Build history of the part. All positions in model axes, mm. Give positions to 0.01 mm unless a question says otherwise; leave off trailing zeros. Write each loop counter-clockwise with the first axis right and the second up, starting at its lowest first coordinate (ties: lowest second). Pieces come first, ordered by that corner, then holes. Notation, with made-up numbers: (16, 64.5) -> (69, 64.5) arc R23 cw to (69, 88.5) -> close; hole circle Ø3 at (-35, 38). An arc over 180 degrees is marked (long way). One line per question, with ' | ' between items. Start each with the question number.
(1) Band-saw the part on A-A, the plane y = -23. Give the cut face in (x, z), and give its area (3 significant figures).
(2) Band-saw the part on B-B, the plane x = -35. Give the cut face in (y, z).
(3) Band-saw the part on D-D, the plane x = -2.5. Give the cut face in (y, z).
(4) Drill centre lines: probe 1 along X at (y, z) = (-30, 0.9); probe 2 along X at (y, z) = (-3, 3.25); probe 3 along Y at (x, z) = (42.5, 3.6). Where is each one in solid material? Low to high. Write a range as from..to.
(5) Band-saw the part on C-C, the plane z = 3. Count the separate pieces of the cut face and the enclosed holes in it, and give its area (3 significant figures).
from build123d import *

# Parameters (mm, degrees)
SKETCH1_R           = 2.1
BOSS_EXTRUDE1_DEPTH = 5
CUT_EXTRUDE1_DEPTH  = 5
SKETCH3_W           = 38.251438616
SKETCH3_H           = 32.766065525
CUT_EXTRUDE2_DEPTH  = 10
BOSS_EXTRUDE2_DEPTH = 5
SKETCH5_W           = 101.856885825
SKETCH5_H           = 15.226385752
CUT_EXTRUDE3_DEPTH  = 10
BOSS_EXTRUDE3_DEPTH = 5
CUT_EXTRUDE4_DEPTH  = 5
SKETCH8_R           = 2.5
SKETCH8_W           = 20
SKETCH8_H           = 40
CUT_EXTRUDE5_DEPTH  = 5
FILLET2_R           = 7


with BuildPart() as part:
    # Sketch1 → Boss-Extrude1 (new body)
    with BuildSketch(Plane.XY):
        Polygon((27.058043777, 13.348752177), (18.058043777, 13.348752177), (18.058043777, 18.348752177), (-18.941956223, 18.348752177), (-18.941956223, 13.348752177), (-27.941956223, 13.348752177), (-27.941956223, 1.348752177), (-27.941956223, -10.651247823), (-63.297295282, -46.006586882), (-51.297295282, -58.006586882), (50.413382836, -58.006586882), (62.413382836, -46.006586882), (27.058043777, -10.651247823), (27.058043777, 1.348752177), align=None)
        with Locations((9.558043777, -11.651247823)):
            Circle(SKETCH1_R, mode=Mode.SUBTRACT)
        with Locations((-10.441956223, -11.651247823)):
            Circle(SKETCH1_R, mode=Mode.SUBTRACT)
        with Locations((-10.441956223, 14.348752177)):
            Circle(SKETCH1_R, mode=Mode.SUBTRACT)
        with Locations((9.558043777, 14.348752177)):
            Circle(SKETCH1_R, mode=Mode.SUBTRACT)
        with BuildLine():
            ThreePointArc((-8.691956223, 1.348752177), (-12.941956223, 5.598752177), (-17.191956223, 1.348752177))
            ThreePointArc((-17.191956223, 1.348752177), (-12.941956223, -2.901247823), (-8.691956223, 1.348752177))
        make_face(mode=Mode.SUBTRACT)
        with BuildLine():
            ThreePointArc((16.308043777, 1.348752177), (12.058043777, 5.598752177), (7.808043777, 1.348752177))
            ThreePointArc((7.808043777, 1.348752177), (12.058043777, -2.901247823), (16.308043777, 1.348752177))
        make_face(mode=Mode.SUBTRACT)
    extrude(amount=BOSS_EXTRUDE1_DEPTH)

    # Sketch2 → Cut-Extrude1 (cut)
    with BuildSketch(Plane(origin=(0, 0, 0), x_dir=(-1, 0, 0), z_dir=(0, 0, -1))):
        with BuildLine():
            Line((-27.058043777, -22.48694002), (-27.058043777, -151.230871916))
            ThreePointArc((-27.058043777, -151.230871916), (0.441956223, -156.858905968), (27.941956223, -151.230871916))
            Line((27.941956223, -151.230871916), (27.941956223, -22.48694002))
            ThreePointArc((27.941956223, -22.48694002), (0.441956223, -16.858905968), (-27.058043777, -22.48694002))
        make_face()
    extrude(amount=-CUT_EXTRUDE1_DEPTH, mode=Mode.SUBTRACT)

    # Sketch3 → Cut-Extrude2 (cut)
    with BuildSketch(Plane(origin=(0, 0, 0), x_dir=(-1, 0, 0), z_dir=(0, 0, -1))):
        with Locations((-46.183763085, -43.921177391)):
            Rectangle(SKETCH3_W, SKETCH3_H)
        with Locations((47.067675531, -43.921177391)):
            Rectangle(SKETCH3_W, SKETCH3_H)
    extrude(amount=-CUT_EXTRUDE2_DEPTH, mode=Mode.SUBTRACT)

    # Sketch4 → Boss-Extrude2 (add)
    with BuildSketch(Plane(origin=(0, 0, 0), x_dir=(-1, 0, 0), z_dir=(0, 0, -1))):
        with BuildLine():
            Line((27.941956223, -10.651247823), (44.828853028, -27.538144628))
            Line((44.828853028, -27.538144628), (50.941956223, -27.538144628))
            Line((50.941956223, -27.538144628), (50.941956223, 27.461855372))
            ThreePointArc((50.941956223, 27.461855372), (49.477490129, 30.997389278), (45.941956223, 32.461855372))
            Line((45.941956223, 32.461855372), (-45.058043777, 32.461855372))
            ThreePointArc((-45.058043777, 32.461855372), (-48.593577683, 30.997389278), (-50.058043777, 27.461855372))
            Line((-50.058043777, 27.461855372), (-50.058043777, -27.538144628))
            Line((-50.058043777, -27.538144628), (-43.944940582, -27.538144628))
            Line((-43.944940582, -27.538144628), (-27.058043777, -10.651247823))
            Line((-27.058043777, -10.651247823), (-27.058043777, 13.348752177))
            Line((-27.058043777, 13.348752177), (-18.058043777, 13.348752177))
            Line((-18.058043777, 13.348752177), (-18.058043777, 18.348752177))
            Line((-18.058043777, 18.348752177), (18.941956223, 18.348752177))
            Line((18.941956223, 18.348752177), (18.941956223, 13.348752177))
            Line((18.941956223, 13.348752177), (27.941956223, 13.348752177))
            Line((27.941956223, 13.348752177), (27.941956223, -10.651247823))
        make_face()
    extrude(amount=-BOSS_EXTRUDE2_DEPTH)

    # Sketch5 → Cut-Extrude3 (cut)
    with BuildSketch(Plane.XY.offset(5)):
        with Locations((-0.013513311, 25.961945053)):
            Rectangle(SKETCH5_W, SKETCH5_H)
    extrude(amount=-CUT_EXTRUDE3_DEPTH, mode=Mode.SUBTRACT)

    # Sketch6 → Boss-Extrude3 (add)
    with BuildSketch(Plane.XY.offset(5)):
        with BuildLine():
            Line((50.058043777, -27.538144628), (27.058043777, -27.538144628))
            Line((27.058043777, -27.538144628), (27.058043777, -22.48694002))
            ThreePointArc((27.058043777, -22.48694002), (-0.441956223, -16.858905968), (-27.941956223, -22.48694002))
            Line((-27.941956223, -22.48694002), (-27.941956223, -27.538144628))
            Line((-27.941956223, -27.538144628), (-50.941956223, -27.538144628))
            Line((-50.941956223, -27.538144628), (-50.941956223, -42.538144628))
            Line((-50.941956223, -42.538144628), (-12.941956223, -42.538144628))
            Line((-12.941956223, -42.538144628), (12.058043777, -42.538144628))
            Line((12.058043777, -42.538144628), (50.058043777, -42.538144628))
            Line((50.058043777, -42.538144628), (50.058043777, -27.538144628))
        make_face()
    extrude(amount=-BOSS_EXTRUDE3_DEPTH)

    # Sketch7 → Cut-Extrude4 (cut)
    with BuildSketch(Plane.XY.offset(5)):
        with BuildLine():
            Line((-27.941956223, -27.962811021), (-27.941956223, -42.538144628))
            Line((-27.941956223, -42.538144628), (27.058043777, -42.538144628))
            Line((27.058043777, -42.538144628), (27.058043777, -27.962811021))
            ThreePointArc((27.058043777, -27.962811021), (-0.441956223, -21.858905968), (-27.941956223, -27.962811021))
        make_face()
    extrude(amount=-CUT_EXTRUDE4_DEPTH, mode=Mode.SUBTRACT)

    # Sketch8 → Cut-Extrude5 (cut)
    with BuildSketch(Plane(origin=(0, 0, 0), x_dir=(-1, 0, 0), z_dir=(0, 0, -1))):
        with Locations((44.521956223, 12.405303775)):
            Circle(SKETCH8_R)
        with Locations((34.361956223, 12.405303775)):
            Circle(SKETCH8_R)
        with Locations((34.361956223, -36.594696225)):
            Circle(SKETCH8_R)
        with Locations((44.521956223, -36.594696225)):
            Circle(SKETCH8_R)
        with Locations((-43.638043777, -36.594696225)):
            Circle(SKETCH8_R)
        with Locations((-33.478043777, -36.594696225)):
            Circle(SKETCH8_R)
        with Locations((-33.478043777, 12.405303775)):
            Circle(SKETCH8_R)
        with Locations((-43.638043777, 12.405303775)):
            Circle(SKETCH8_R)
        with Locations((39.441956223, -12.094696225)):
            Rectangle(SKETCH8_W, SKETCH8_H)
        with Locations((-38.558043777, -12.094696225)):
            Rectangle(SKETCH8_W, SKETCH8_H)
    extrude(amount=-CUT_EXTRUDE5_DEPTH, mode=Mode.SUBTRACT)

    # Fillet2
    fillet2_edges = [part.edges().sort_by_distance(p)[0] for p in [
        (50.058043777, 18.348752177, 2.5),
        (-50.941956223, 18.348752177, 2.5),
        (50.058043777, -42.538144628, 2.5),
        (-50.941956223, -42.538144628, 2.5),
    ]]
    fillet(fillet2_edges, radius=FILLET2_R)


solid = part.part
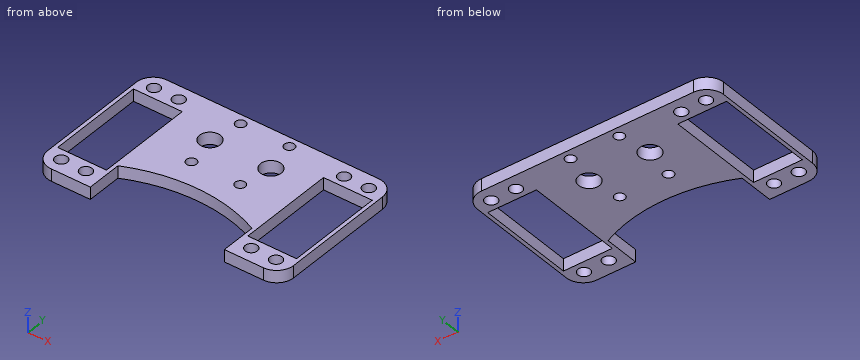
Results:
1) outline: (-50.94, 0) -> (-49.44, 0) -> (-49.44, 5) -> (-50.94, 5) -> close; (-29.44, 0) -> (-12.57, 0) -> (-12.57, 5) -> (-29.44, 5) -> close; (11.68, 0) -> (28.56, 0) -> (28.56, 5) -> (11.68, 5) -> close; (48.56, 0) -> (50.06, 0) -> (50.06, 5) -> (48.56, 5) -> close | area: 184 mm²
2) outline: (-42.54, 0) -> (-39.01, 0) -> (-39.01, 5) -> (-42.54, 5) -> close; (-34.18, 0) -> (-32.09, 0) -> (-32.09, 5) -> (-34.18, 5) -> close; (7.91, 0) -> (9.99, 0) -> (9.99, 5) -> (7.91, 5) -> close; (14.82, 0) -> (18.35, 0) -> (18.35, 5) -> (14.82, 5) -> close
3) outline: (-21.89, 0) -> (18.35, 0) -> (18.35, 5) -> (-21.89, 5) -> close
4) probe 1: x = -50.94..-49.44, -29.44..-27.94, 27.06..28.56, 48.56..50.06 | probe 2: x = -50.94..-49.44, -29.44..28.56, 48.56..50.06 | probe 3: y = -42.54..-38.82, -34.37..-32.09, 7.91..10.18, 14.63..18.35
5) separate pieces: 1 | enclosed holes: 16 | area: 3,150 mm²
